The model under review builds one solid part; all positions refer to its coordinate system, in mm. A direction names the side the tool comes from. Coordinates: 2 decimals unless noted, no trailing zeros. Order: outer loops, then holes, each group sorted by start corner. A loop starts at its lowest first (then second) coordinate and runs counter-clockwise, first axis right, second up. Notation, with made-up numbers: M 11,13 L 43,13 A24 cw 43,30 Z; hole C 16.25,-22.5 d4. An arc over 180 degrees is marked long. Answer in a Markdown table with one row per item.
from build123d import *

# Parameters (mm, degrees)
SKETCH1_W           = 34
SKETCH1_H           = 20
BOSS_EXTRUDE1_DEPTH = 3
FILLET1_R           = 3
SKETCH2_W           = 14
SKETCH2_H           = 20
BOSS_EXTRUDE2_DEPTH = 20
CUT_EXTRUDE1_DEPTH  = 35.899856733
CHAMFER1_SIZE       = 1
SKETCH4_R           = 2.2
CUT_EXTRUDE2_DEPTH  = 29.08914381
SKETCH5_R           = 1.7
CUT_EXTRUDE3_DEPTH  = 39.340579025
FILLET2_R           = 2
CUT_EXTRUDE4_DEPTH  = 2.5
SKETCH7_R           = 2.75
CUT_EXTRUDE5_DEPTH  = 3
SKETCH8_R           = 2.2
CUT_EXTRUDE6_DEPTH  = 31.298514848
SKETCH9_R           = 4.5
CUT_EXTRUDE7_DEPTH  = 21


with BuildPart() as part:
    # Sketch1 → Boss-Extrude1 (new body)
    with BuildSketch(Plane.XY):
        Rectangle(SKETCH1_W, SKETCH1_H)
    extrude(amount=BOSS_EXTRUDE1_DEPTH)

    # Fillet1
    fillet1_edges = [part.edges().sort_by_distance(p)[0] for p in [
        (17, -10, 1.5),
        (-17, -10, 1.5),
        (-17, 10, 1.5),
        (17, 10, 1.5),
    ]]
    fillet(fillet1_edges, radius=FILLET1_R)

    # Sketch2 → Boss-Extrude2 (add)
    with BuildSketch(Plane.XY.offset(3)):
        with Locations((5, 0)):
            Rectangle(SKETCH2_W, SKETCH2_H)
    extrude(amount=BOSS_EXTRUDE2_DEPTH)

    # Sketch3 → Cut-Extrude1 (cut, through all)
    with BuildSketch(Plane(origin=(0, 10, 0), x_dir=(1, 0, 0), z_dir=(0, 1, 0))):
        with BuildLine():
            Line((4.5, -16.119769411), (4.5, -23))
            Line((4.5, -23), (5.5, -23))
            Line((5.5, -23), (5.5, -16.119769411))
            ThreePointArc((5.5, -16.119769411), (5, -7.85), (4.5, -16.119769411))
        make_face()
    extrude(amount=-CUT_EXTRUDE1_DEPTH, mode=Mode.SUBTRACT)

    # Chamfer1
    chamfer1_edges = [part.edges().sort_by_distance(p)[0] for p in [
        (5, -10, 7.85),
        (5, 10, 7.85),
    ]]
    chamfer(chamfer1_edges, length=CHAMFER1_SIZE)

    # Sketch4 → Cut-Extrude2 (cut, through all)
    with BuildSketch(Plane.XY.offset(3)):
        with Locations((-9.5, 0)):
            Circle(SKETCH4_R)
    extrude(amount=-CUT_EXTRUDE2_DEPTH, mode=Mode.SUBTRACT)

    # Sketch5 → Cut-Extrude3 (cut, through all)
    with BuildSketch(Plane(origin=(12, 0, 0), x_dir=(0, 0, -1), z_dir=(1, 0, 0))):
        with Locations(Location((-19.5, 5, 0), (0, 0, 90))):
            Circle(SKETCH5_R)
        with Locations(Location((-19.5, -5, 0), (0, 0, 90))):
            Circle(SKETCH5_R)
    extrude(amount=-CUT_EXTRUDE3_DEPTH, mode=Mode.SUBTRACT)

    # Fillet2
    # the kernel refuses this fillet: 2 mm, written as the material it takes off along each edge
    with BuildSketch(Plane(origin=(12, -15, 23), x_dir=(-1, 0, 0), z_dir=(0, 1, 0)), Plane(origin=(-2, 15, 23), x_dir=(1, 0, 0), z_dir=(0, -1, 0))) as fillet2_piece_1:
        with BuildLine():
            CenterArc((FILLET2_R, -FILLET2_R), FILLET2_R, 90, 90)
            Line((0, -FILLET2_R), (0, 0))
            Line((0, 0), (FILLET2_R, 0))
        make_face()
    extrude(amount=30, mode=Mode.SUBTRACT)

    # Sketch6 → Cut-Extrude4 (cut)
    with BuildSketch(Plane(origin=(12, 0, 0), x_dir=(0, 0, -1), z_dir=(1, 0, 0))):
        Polygon((-16.7, 3.383419246), (-16.7, 6.616580754), (-19.5, 8.233161507), (-22.3, 6.616580754), (-22.3, 3.383419246), (-19.5, 1.766838493), align=None)
        Polygon((-16.7, -3.383419246), (-19.5, -1.766838493), (-22.3, -3.383419246), (-22.3, -6.616580754), (-19.5, -8.233161507), (-16.7, -6.616580754), align=None)
    extrude(amount=-CUT_EXTRUDE4_DEPTH, mode=Mode.SUBTRACT)

    # Sketch7 → Cut-Extrude5 (cut)
    with BuildSketch(Plane.ZY.offset(2)):
        with Locations(Location((19.5, 5, 0), (0, 0, 270))):
            Circle(SKETCH7_R)
        with Locations(Location((19.5, -5, 0), (0, 0, 270))):
            Circle(SKETCH7_R)
    extrude(amount=-CUT_EXTRUDE5_DEPTH, mode=Mode.SUBTRACT)

    # Sketch8 → Cut-Extrude6 (cut, through all)
    with BuildSketch(Plane.XY.offset(23)):
        with Locations((5, 0)):
            Circle(SKETCH8_R)
    extrude(amount=-CUT_EXTRUDE6_DEPTH, mode=Mode.SUBTRACT)

    # Sketch9 → Cut-Extrude7 (cut)
    with BuildSketch(Plane.XY.offset(23)):
        with Locations((5, 0)):
            Circle(SKETCH9_R)
    extrude(amount=-CUT_EXTRUDE7_DEPTH, mode=Mode.SUBTRACT)


solid = part.part
(1) Take a section at C-C (x = -9.5). Write out the cut boundary in (y, z), then the cut area to 3 significant figures.
Report:
| item | result |
|---|---|
| outline | M -10,0 L -2.2,0 L -2.2,3 L -10,3 Z; M 2.2,0 L 10,0 L 10,3 L 2.2,3 Z |
| area | 46.8 mm^2 |
(2) Take a section at B-B (x = 5). Write out the cut boundary in (y, z).
Report:
| item | result |
|---|---|
| outline | M -10,0 L -2.2,0 L -2.2,2 L -4.5,2 L -4.5,7.85 L -9,7.85 L -10,6.85 Z; M 2.2,0 L 10,0 L 10,6.85 L 9,7.85 L 4.5,7.85 L 4.5,2 L 2.2,2 Z |
(3) Insertion check: P1, Ø6, axis at y = -4.5, z = 20, coming from the -X side; P2, Ø4.5, axis at y = -5, z = 19.5, coming from the -X side; P3, Ø8, axis at x = -11, y = 5, coming from the -Z side; P4, Ø3, axis at y = 3.5, z = 18.5, coming from the +X side. Each pin has a flat end and moves straight along its axis. Give the tip position at first contact, or say it passes through.
Report:
| item | result |
|---|---|
| P1 | x = -2 |
| P2 | x = 1 |
| P3 | z = 0 |
| P4 | x = 12 |
(4) To check wall thickness, follow line 1 (Y direction, x = -9.5, z = 1.15); line 2 (Z direction, x = 1.75, y = -5); line 3 (Y direction, x = 3.35, z = 19.5). State the ranges of each line that lie inside material, in increasing order. Write a range as [from, to].
Report:
| item | result |
|---|---|
| line 1 | [-10, -2.2], [2.2, 10] |
| line 2 | [0, 9.42], [14.58, 17.8], [21.2, 23] |
| line 3 | [-10, -6.7], [6.7, 10] |
(5) The part is to be moulded in two halves that separate along Z. For faces 1 (the cylindrical face through (-0.521, 5.596, 16.815)), 2 (the flat face through (0.2, 0.1, 23)), 3 (the flat face through (5.5, 8, 20)), 4 (the flat face through (10.768, -2.586, 18.08)), say which applies: +Z half, -Z half, draft (parallel to the pull), parting line (faces both ways), or undercut.
Report:
| item | result |
|---|---|
| face 1 | undercut |
| face 2 | +Z half |
| face 3 | draft |
| face 4 | undercut |
(6) Machinability: for faces 5 (the flat face through (11, 5, 16.7)), 6 (the cylindrical face through (9.292, 1.352, 12.647)), 7 (the flat face through (9.7, 0.1, 23)), 8 (the flat face through (1, -7, 20)), 9 (the flat face through (-2, 0, 12)), which of the approach directions +Z, -Z, +X, -X, +Y, -Y give a long, thin tool a straight path to every point of the face, cutting with its end or side? Answer none if there is none.
Report:
| item | result |
|---|---|
| face 5 | +X |
| face 6 | +Z |
| face 7 | +Z, +X, -X, +Y, -Y |
| face 8 | -X |
| face 9 | +Z, -X, +Y, -Y |
(7) Take a section at A-A (y = 0). Write out the cut boundary in (x, z), then the cut area to 3 significant figures.
Report:
| item | result |
|---|---|
| outline | M -17,0 L -11.7,0 L -11.7,3 L -17,3 Z; M -7.3,0 L 2.8,0 L 2.8,2 L 0.5,2 L 0.5,23 L 0,23 A2 ccw -2,21 L -2,3 L -7.3,3 Z; M 7.2,0 L 17,0 L 17,3 L 12,3 L 12,21 A2 ccw 10,23 L 9.5,23 L 9.5,2 L 7.2,2 Z |
| area | 169 mm^2 |
(8) Take a section at D-D (y = -6). Write out the cut boundary in (x, z).
Report:
| item | result |
|---|---|
| outline | M -17,0 L 17,0 L 17,3 L 12,3 L 12,16.7 L 9.5,16.7 L 9.5,18.13 L 5.5,18.13 L 5.5,16.12 A4.15 cw long 4.5,16.12 L 4.5,18.13 L 1,18.13 L 1,16.94 L -2,16.94 L -2,3 L -17,3 Z; M -1.69,22.06 L 1,22.06 L 1,20.87 L 4.5,20.87 L 4.5,23 L 0,23 A2 ccw Z; M 5.5,20.87 L 9.5,20.87 L 9.5,22.3 L 11.52,22.3 A2 ccw 10,23 L 5.5,23 Z |
